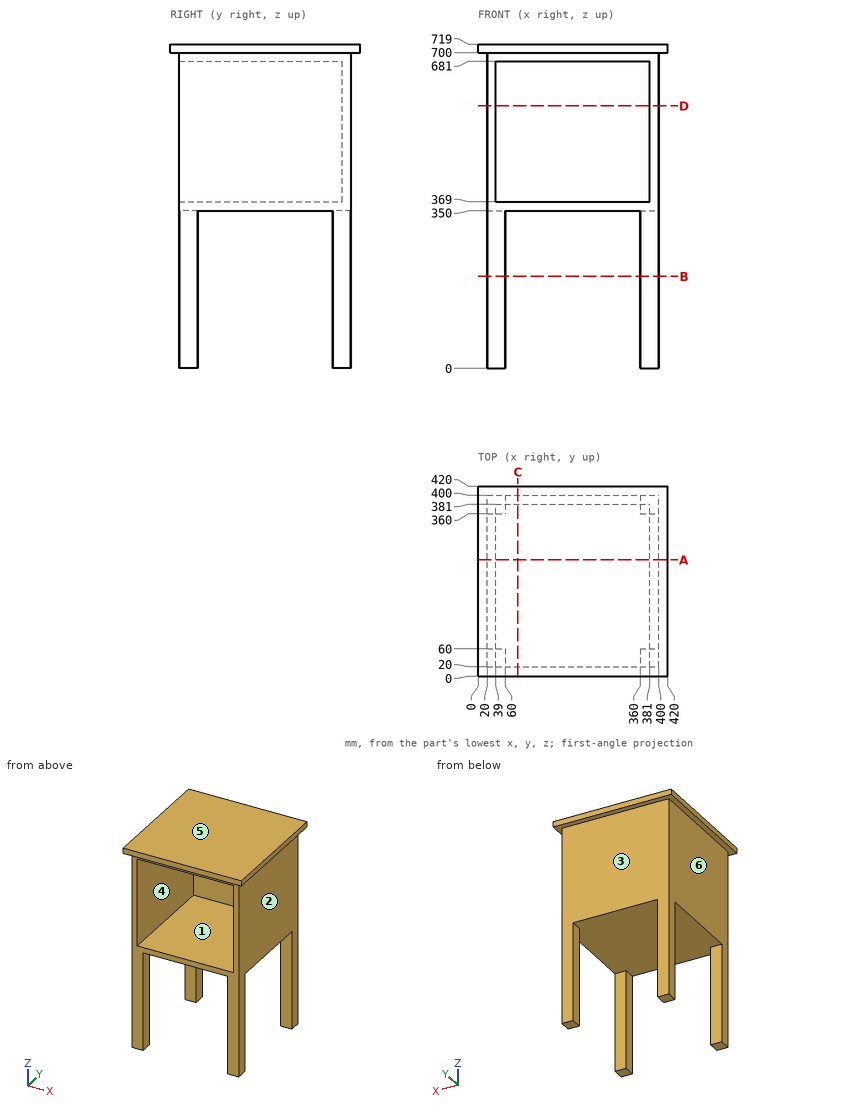
Study the drawing (mm; zero at the part's minimum x, y, z) and answer. A direction names the side the tool comes from. Coordinates: 2 decimals unless noted, no trailing zeros. Write each loop counter-clockwise with the first axis right and the second up, starting at its lowest first coordinate (ties: lowest second). Pieces come first, ordered by that corner, then holes. Notation, with made-up numbers: M -18.5,71 L 7.5,71 A5 cw 7.5,80 Z; hole C 63.25,0.25 d9. An arc over 180 degrees is marked long. Write each question's results on one line, items separated by ' | '.
Item 1: For a pull along Z with two mould halves and no side action, classify the marked faces 4, 5 and 6 as released by +Z, released by -Z, zero draft, split by the parting line, or undercut.
Answer below:
face 4: undercut | face 5: released by +Z | face 6: zero draft
Item 2: The part is cut by section B-B on z = 204. Determine the outline of the cut face in (x, y).
Answer below:
outline: M 20,20 L 60,20 L 60,60 L 20,60 Z; M 20,360 L 60,360 L 60,400 L 20,400 Z; M 360,20 L 400,20 L 400,60 L 360,60 Z; M 360,360 L 400,360 L 400,400 L 360,400 Z
Item 3: The part is cut by section A-A on y = 257.5. Determine the outline of the cut face in (x, z).
Answer below:
outline: M 0,700 L 20,700 L 20,350 L 400,350 L 400,700 L 420,700 L 420,719 L 0,719 Z; hole M 39,369 L 381,369 L 381,681 L 39,681 Z
Item 4: Given P1, Ø20, axis at x = 45.5, z = 187.5, coming from the -Y side; P2, Ø4, axis at x = 125.5, z = 605, coming from the -Y side; P3, Ø12, axis at y = 377.5, z = 226.5, coming from the -X side, each flat-ended and moving along its own axis, determine where each tip first touches the part or whether it passes through.
Answer below:
P1: y = 20 | P2: y = 381 | P3: x = 20
Item 5: Consider probe 1 along Z at (x, y) = (198, 59); probe 2 along X at (y, z) = (30, 66); probe 3 along X at (y, z) = (201, 596.5). Determine where each line is inside the solid, lowest interval first. Write a range as [from, to].
Answer below:
probe 1: [350, 369], [681, 719] | probe 2: [20, 60], [360, 400] | probe 3: [20, 39], [381, 400]
Item 6: Which of the six approach directions +Z, -Z, +X, -X, +Y, -Y give full straight-line access (tool end or side, diameter ignored) to the marked faces 1, 2 and 3?
Answer below:
face 1: -Y | face 2: -Z, +X, +Y, -Y | face 3: -Z, +X, -X, +Y
Item 7: The part is cut by section C-C on x = 88.5. Determine the outline of the cut face in (y, z).
Answer below:
outline: M 0,700 L 20,700 L 20,681 L 381,681 L 381,369 L 20,369 L 20,350 L 400,350 L 400,700 L 420,700 L 420,719 L 0,719 Z
Item 8: The part is cut by section D-D on z = 582. Determine the outline of the cut face in (x, y).
Answer below:
outline: M 20,20 L 39,20 L 39,381 L 381,381 L 381,20 L 400,20 L 400,400 L 20,400 Z
